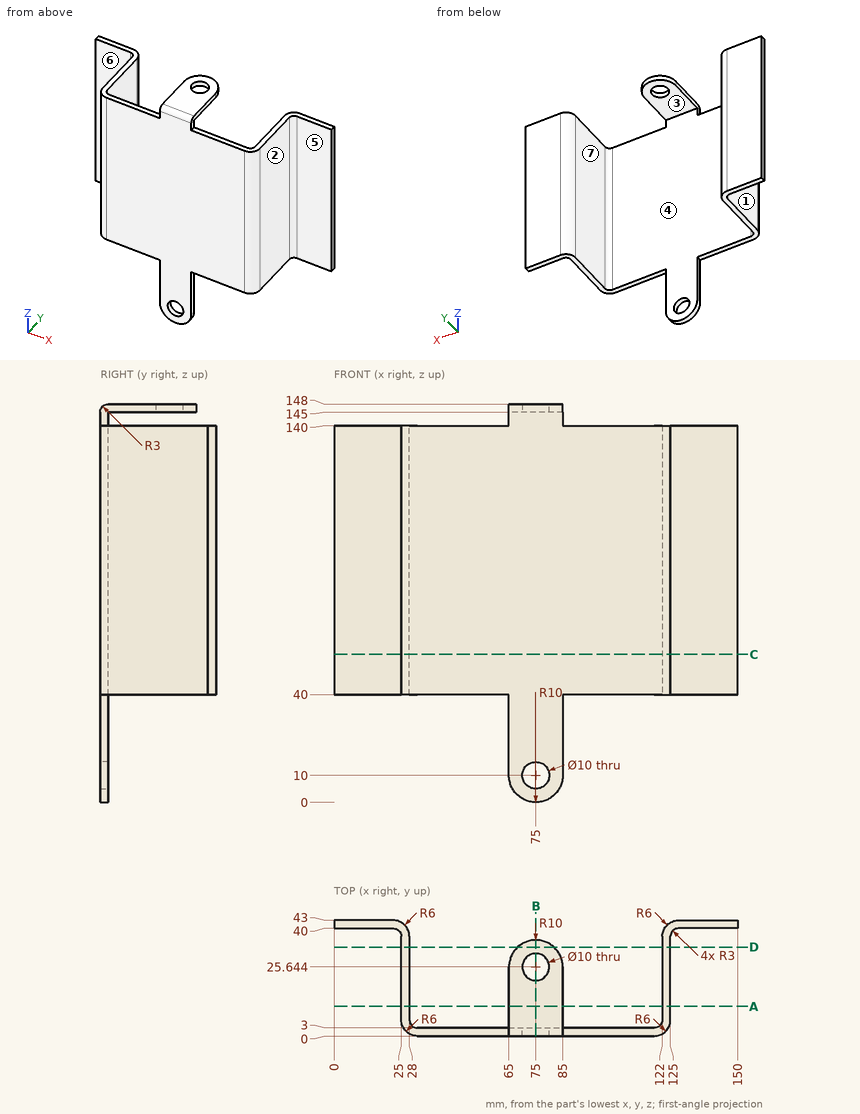
Design review of the part shown in the three views and the two pictorial views. Dimensions are in mm from the part's minimum x, y and z. A direction names the side the tool comes from. Give positions to 0.01 mm unless a question says otherwise; leave off trailing zeros. Order: outer loops, then holes, each group sorted by start corner. A loop starts at its lowest first (then second) coordinate and runs counter-clockwise, first axis right, second up. Notation, with made-up numbers: M 26,28.5 L 44,28.5 A15 ccw 44,52.5 Z; hole C -35,25.5 d10. An arc over 180 degrees is marked long. Answer in a Markdown table with one row per item. Add a question column.
(1) Consider section A-A on y = 11. State the section outline as (x, z) points.
(2) Consider section C-C on z = 55. State the section outline as (x, y) points.
(3) For the marked faces 5, 6 and 7, list the 3-axis set-ups (+Z, -Z, +X, -X, +Y, -Y) from which the entire face can be reached by the end or side of a thin tool; tool diameter is ignored.
(4) For pin 1 (3 mm diameter, centred on x = 77.5, z = 90, fed in from +Y); pin 2 (4 mm diameter, centred on y = 15.5, z = 52, fed in from -X); pin 3 (6 mm diameter, centred on x = 25, y = 9.5, fed in from -Z), all flat-tipped, find the tip position at first contact; note any pin that passes through.
(5) Consider section B-B on x = 75. State the section outline as (y, z) points.
(6) Wall thickness on probe 1 along X at (y, z) = (24.5, 78); probe 2 along X at (y, z) = (1.55, 10); probe 3 along Y at (x, z) = (66.5, 15): over which ranges is each line inside the solid? List them lowest first. Write a range as [from, to].
(7) Mouldability with a two-part tool opening along X and no side actions: class the marked faces 1, 2, 3 and 4 as +X half, -X half, draft (parallel to the pull), parting line (faces both ways), or undercut.
(8) Consider section D-D on y = 33. State the section outline as (x, z) points.
Evaluation:
| question | item | result |
|---|---|---|
| 1 | outline | M 25,40 L 28,40 L 28,140 L 25,140 Z; M 65,145 L 85,145 L 85,148 L 65,148 Z; M 122,40 L 125,40 L 125,140 L 122,140 Z |
| 2 | outline | M 0,40 L 22,40 A3 cw 25,37 L 25,6 A6 ccw 31,0 L 119,0 A6 ccw 125,6 L 125,37 A3 cw 128,40 L 150,40 L 150,43 L 128,43 A6 ccw 122,37 L 122,6 A3 cw 119,3 L 31,3 A3 cw 28,6 L 28,37 A6 ccw 22,43 L 0,43 Z |
| 3 | face 5 | +Z, -Z, +X, -Y |
| 3 | face 6 | +Z, -Z, -X, -Y |
| 3 | face 7 | +Z, -Z, +Y |
| 4 | pin 1 | stops at y = 3 |
| 4 | pin 2 | stops at x = 25 |
| 4 | pin 3 | stops at z = 40 |
| 5 | outline | M 0,0 L 3,0 L 3,5 L 0,5 Z; M 0,15 L 3,15 L 3,145 L 20.64,145 L 20.64,148 L 3,148 A3 ccw 0,145 Z; M 30.64,145 L 35.64,145 L 35.64,148 L 30.64,148 Z |
| 6 | probe 1 | x = [25, 28], [122, 125] |
| 6 | probe 2 | x = [65, 70], [80, 85] |
| 6 | probe 3 | y = [0, 3] |
| 7 | face 1 | -X half |
| 7 | face 2 | +X half |
| 7 | face 3 | draft |
| 7 | face 4 | undercut |
| 8 | outline | M 25,40 L 28,40 L 28,140 L 25,140 Z; M 68.23,145 L 81.77,145 L 81.77,148 L 68.23,148 Z; M 122,40 L 125,40 L 125,140 L 122,140 Z |
